Check sheet for the modelled part. Datum: model origin and axes. Units: mm. Give positions to 0.01 mm unless a question says otherwise; leave off trailing zeros. Order: outer loops, then holes, each group sorted by start corner. A loop starts at its lowest first (then second) coordinate and runs counter-clockwise, first axis right, second up.
from build123d import *

# Parameters (mm, degrees)
SKETCH1_R           = 76.2
SKETCH1_R_2         = 49.149
EXTRUDE_THIN1_DEPTH = 19.05
SKETCH2_R           = 4.2164
CUT_EXTRUDE3_DEPTH  = 20.05
CIRPATTERN1_COUNT   = 16


with BuildPart() as part:
    # Sketch1 → Extrude-Thin1 (new body)
    with BuildSketch(Plane.XY):
        Circle(SKETCH1_R)
        Circle(SKETCH1_R_2, mode=Mode.SUBTRACT)
    extrude(amount=EXTRUDE_THIN1_DEPTH)

    # Sketch2 → Cut-Extrude3 (cut, through all)
    with BuildSketch(Plane.XY):
        with Locations((0, 65.151)):
            Circle(SKETCH2_R)
    cut_extrude3 = extrude(amount=CUT_EXTRUDE3_DEPTH, mode=Mode.SUBTRACT)

    # CirPattern1: Cut-Extrude3 ×16 about axis
    cirpattern1_axis = Axis((0, 0, 0), (0, 0, 1))
    for i in range(1, CIRPATTERN1_COUNT):
        add(cut_extrude3.rotate(cirpattern1_axis, i * 360 / CIRPATTERN1_COUNT), mode=Mode.SUBTRACT)


solid = part.part
1) Section check A-A, the plane y = 0. Record the cut outline in (x, z).
Recorded:
outline: (-76.2, 0) - (-69.37, 0) - (-69.37, 19.05) - (-76.2, 19.05) - close; (-60.93, 0) - (-49.15, 0) - (-49.15, 19.05) - (-60.93, 19.05) - close; (49.15, 0) - (60.93, 0) - (60.93, 19.05) - (49.15, 19.05) - close; (69.37, 0) - (76.2, 0) - (76.2, 19.05) - (69.37, 19.05) - close
2) Section check D-D, the plane y = -34. Record the cut outline in (x, z).
Recorded:
outline: (-68.19, 0) - (-35.49, 0) - (-35.49, 19.05) - (-68.19, 19.05) - close; (35.49, 0) - (68.19, 0) - (68.19, 19.05) - (35.49, 19.05) - close
3) Material ranges on L1, parallel to Y at x = 0, z = 6.25; L2, parallel to X at y = -3, z = 13.75; L3, parallel to Y at x = -23.5, z = 2, recorded low to high.
Recorded:
L1: y = -76.2 to -69.37, -60.93 to -49.15, 49.15 to 60.93, 69.37 to 76.2
L2: x = -76.14 to -68.11, -62.19 to -49.06, 49.06 to 62.19, 68.11 to 76.14
L3: y = -72.49 to -64.16, -56.23 to -43.17, 43.17 to 56.23, 64.16 to 72.49
4) Section check C-C, the plane z = 13.75. State how many separate pieces and enclosed holes the cut face has, then the cut area to 3 significant figures.
Recorded:
separate pieces: 1
enclosed holes: 17
area: 9,760 mm2
5) Depth check by flat-ended pin: pin 1 Ø5 at (y, z) = (-14.5, 3) entering from +X; pin 2 Ø5 at (x, z) = (-59, 6.5) entering from -Y; pin 3 Ø6 at (y, z) = (-35, 11) entering from -X. Enter the tip coordinate at first touch or a pass-through.
Recorded:
pin 1: stops at x = 75.25
pin 2: stops at y = -51.13
pin 3: stops at x = -69.16
6) Draft check along X on faces 1 (the face through (-60.47, -46.367, 9.392)), 2 (the face through (0.55, -69.33, 9.39)), 3 (the face through (-1, -50, 0)), 4 (the face through (-63.844, -27.039, 9.392)). Enter one of: +X half, -X half, draft (parallel to the pull), parting line (faces both ways), or undercut.
Recorded:
face 1: parting line
face 2: undercut
face 3: draft
face 4: undercut
